Design review of the part built by this model. Coordinates are the model's own, in mm. A direction names the side the tool comes from. Round coordinates to 2 decimals unless told otherwise and drop trailing zeros. Write each loop counter-clockwise with the first axis right and the second up, starting at its lowest first coordinate (ties: lowest second). Pieces come first, ordered by that corner, then holes. Notation, with made-up numbers: (51, -36) -> (79, -36) arc R31 ccw to (79, -6) -> close; hole circle Ø11 at (-18.5, -11). An arc over 180 degrees is marked (long way). One line per question, with ' | ' between items. Start each with the question number.
1) Consider section D-D (z = -4). Give the boundary of the cut face in (x, y), then the cut area to 3 significant figures.
2) Mouldability with a two-part tool opening along X and no side actions: class faces 1 (the cylindrical face through (1, -2, 0)), 2 (the flat face through (11, -43, 10.75)), 3 (the flat face through (7.75, -43, -9)), 4 (the flat face through (14.75, -44.3, 9.7)) as +X half, -X half, draft (parallel to the pull), parting line (faces both ways), or undercut.
3) Consider section A-A (y = 2.4). Give the boundary of the cut face in (x, z), then the cut area to 3 significant figures.
4) Consider section B-B (x = 20). Give the boundary of the cut face in (y, z), then the cut area to 3 significant figures.
5) For probe 1 along Y at (x, z) = (11.25, -0.2); probe 2 along Y at (x, z) = (11.25, 2.5); probe 3 along X at (y, z) = (-11, -2.5), list the stretches that pass through material, from the lowest coordinate up.
6) Consider section C-C (y = -39). Give the boundary of the cut face in (x, z).
7) Insertion check: pin 1 Ø10 at (x, y) = (18.5, -11.5) entering from -Z; pin 2 Ø2 at (x, z) = (15, 0.5) entering from -Y; pin 3 Ø1.5 at (x, y) = (12.5, 3) entering from +Z. Each pin has a flat end and moves straight along its axis. Give the tip position at first contact, or say it passes through.
8) For faces 5 (the flat face through (11.2, -41.5, 7.6)), 6 (the flat face through (11, -44, -10)), 7 (the flat face through (11, -37, -1)), 8 (the flat face through (11.3, -37, 8.5)), 9 (the flat face through (11, -18, 9.4)), list the 3-axis set-ups (+Z, -Z, +X, -X, +Y, -Y) from which the entire face can be reached by the end or side of a thin tool; tool diameter is ignored.
```python
from build123d import *

# Parameters (mm, degrees)
CROQUIS2_R              = 1.5
SALIENTE_EXTRUIR1_DEPTH = 9.4
CROQUIS3_W              = 5
CROQUIS3_H              = 5
CROQUIS3_R              = 1.4
SALIENTE_EXTRUIR2_DEPTH = 1.5
SALIENTE_EXTRUIR3_DEPTH = 12
CROQUIS6_W              = 7
CROQUIS6_H              = 2.5
CORTAR_EXTRUIR1_DEPTH   = 57.687741179
SALIENTE_EXTRUIR4_START = 7.75
SALIENTE_EXTRUIR4_DEPTH = 7
CROQUIS8_R              = 2.7
CORTAR_EXTRUIR2_DEPTH   = 58.737964114


with BuildPart() as part:
    # Croquis2 → Saliente-Extruir1 (new, symmetric)
    with BuildSketch(Plane.XY):
        with BuildLine():
            Line((5, 0), (17.5, 0))
            ThreePointArc((17.5, 0), (21.035533906, -1.464466094), (22.5, -5))
            Line((22.5, -5), (22.5, -37))
            Line((22.5, -37), (0, -37))
            Line((0, -37), (0, -5))
            ThreePointArc((0, -5), (1.464466094, -1.464466094), (5, 0))
        make_face()
        with Locations((2.5, -31.8)):
            Circle(CROQUIS2_R, mode=Mode.SUBTRACT)
        with Locations((20, -31.8)):
            Circle(CROQUIS2_R, mode=Mode.SUBTRACT)
    extrude(amount=SALIENTE_EXTRUIR1_DEPTH, both=True)

    # Croquis3 → Saliente-Extruir2 (add, symmetric)
    with BuildSketch(Plane.XY):
        with Locations((11.25, 2.5)):
            Rectangle(CROQUIS3_W, CROQUIS3_H)
        with Locations((11.25, 2.4)):
            Circle(CROQUIS3_R, mode=Mode.SUBTRACT)
    extrude(amount=SALIENTE_EXTRUIR2_DEPTH, both=True)

    # Croquis5 → Saliente-Extruir3 (add)
    with BuildSketch(Plane.XZ.offset(37)):
        with BuildLine():
            Line((18.75, -9.4), (3.75, -9.4))
            ThreePointArc((3.75, -9.4), (0, -0.65), (3.75, 8.1))
            Line((3.75, 8.1), (18.75, 8.1))
            ThreePointArc((18.75, 8.1), (22.5, -0.65), (18.75, -9.4))
        make_face()
        with BuildLine():
            Line((4.160090451, 7.1), (18.339909549, 7.1))
            ThreePointArc((18.339909549, 7.1), (21.5, -0.65), (18.339909549, -8.4))
            Line((18.339909549, -8.4), (4.160090451, -8.4))
            ThreePointArc((4.160090451, -8.4), (1, -0.65), (4.160090451, 7.1))
        make_face(mode=Mode.SUBTRACT)
    extrude(amount=SALIENTE_EXTRUIR3_DEPTH)

    # Croquis6 → Cortar-Extruir1 (cut, through all)
    with BuildSketch(Plane.XY.offset(8.1)):
        with Locations((11.25, -42.75)):
            Rectangle(CROQUIS6_W, CROQUIS6_H)
    extrude(amount=-CORTAR_EXTRUIR1_DEPTH, mode=Mode.SUBTRACT)

    # Croquis7 → Saliente-Extruir4 (add)
    with BuildSketch(Plane(origin=(0, 0, 0), x_dir=(0, 0, -1), z_dir=(1, 0, 0)).offset(SALIENTE_EXTRUIR4_START)):
        Polygon((-8.1, -44), (-10.75, -44), (-10.75, -42.5), (-11.25, -42.5), (-11.25, -44.444570011), (-8.1, -45), align=None)
    saliente_extruir4 = extrude(amount=SALIENTE_EXTRUIR4_DEPTH)

    # Simetría1: Saliente-Extruir4 across plane
    add(saliente_extruir4.mirror(Plane(origin=(0, 0, -0.65), x_dir=(1, 0, 0), z_dir=(0, 0, -1))))

    # Croquis8 → Cortar-Extruir2 (cut, through all)
    with BuildSketch(Plane(origin=(0, 0, -9.4), x_dir=(-1, 0, 0), z_dir=(0, 0, -1))):
        with Locations((-11.25, -11.2)):
            Circle(CROQUIS8_R)
    extrude(amount=-CORTAR_EXTRUIR2_DEPTH, mode=Mode.SUBTRACT)


solid = part.part
```
From the geometry:
1) outline: (0, -37) -> (0.47, -37) -> (0.47, -49) -> (1.52, -49) -> (1.52, -37) -> (20.98, -37) -> (20.98, -49) -> (22.03, -49) -> (22.03, -37) -> (22.5, -37) -> (22.5, -5) arc R5 ccw to (17.5, 0) -> (5, 0) arc R5 ccw to (0, -5) -> close; hole circle Ø3 at (2.5, -31.8); hole circle Ø5.4 at (11.25, -11.2); hole circle Ø3 at (20, -31.8) | area: 810 mm2
2) face 1: -X half | face 2: draft | face 3: undercut | face 4: +X half
3) outline: (8.75, -1.5) -> (9.85, -1.5) -> (9.85, 1.5) -> (8.75, 1.5) -> close; (12.65, -1.5) -> (13.75, -1.5) -> (13.75, 1.5) -> (12.65, 1.5) -> close | area: 6.60 mm2
4) outline: (-49, -8.01) -> (-37, -8.01) -> (-37, -9.4) -> (-33.3, -9.4) -> (-33.3, 9.4) -> (-37, 9.4) -> (-37, 6.71) -> (-49, 6.71) -> (-49, 4.92) -> (-37, 4.92) -> (-37, -6.22) -> (-49, -6.22) -> close; (-30.3, -9.4) -> (-0.67, -9.4) -> (-0.67, 9.4) -> (-30.3, 9.4) -> close | area: 670 mm2
5) probe 1: y = -37 to -13.9, -8.5 to 1, 3.8 to 5 | probe 2: y = -37 to -13.9, -8.5 to 0 | probe 3: x = 0 to 8.56, 13.94 to 22.5
6) outline: (3.75, -9.4) -> (18.75, -9.4) arc R12.08 ccw to (18.75, 8.1) -> (3.75, 8.1) arc R12.08 ccw to start; hole (4.16, -8.4) -> (18.34, -8.4) arc R11.08 ccw to (18.34, 7.1) -> (4.16, 7.1) arc R11.08 ccw to start
7) pin 1: stops at z = -9.4 | pin 2: stops at y = -37 | pin 3: stops at z = 1.5
8) face 5: +Z, -Z | face 6: none | face 7: -Y | face 8: +Z | face 9: +Z, +X, -X, +Y
